from build123d import *

# Parameters (mm, degrees)
SKETCH7_R           = 50
BOSS_EXTRUDE3_DEPTH = 124.4
SKETCH8_R           = 37.5
CUT_EXTRUDE3_DEPTH  = 56
SKETCH9_R           = 32.5
CUT_EXTRUDE4_DEPTH  = 69.4
SKETCH10_W          = 250
SKETCH10_H          = 100
BOSS_EXTRUDE4_DEPTH = 15
SKETCH11_R          = 37.5
CUT_EXTRUDE5_DEPTH  = 15
SKETCH12_R          = 15
BOSS_EXTRUDE5_DEPTH = 328
LPATTERN1_COUNT     = 2
LPATTERN1_PITCH     = 180
SKETCH13_W          = 250
SKETCH13_H          = 100
BOSS_EXTRUDE6_DEPTH = 15
SKETCH15_R          = 20
CUT_EXTRUDE6_DEPTH  = 15


with BuildPart() as part:
    # Sketch7 → Boss-Extrude3 (new body)
    with BuildSketch(Plane.XY):
        with Locations((15.572802758, -20.527785454)):
            Circle(SKETCH7_R)
    extrude(amount=BOSS_EXTRUDE3_DEPTH)

    # Sketch8 → Cut-Extrude3 (cut)
    with BuildSketch(Plane.XY.offset(124.4)):
        with Locations((15.572802758, -20.527785454)):
            Circle(SKETCH8_R)
    extrude(amount=-CUT_EXTRUDE3_DEPTH, mode=Mode.SUBTRACT)

    # Sketch9 → Cut-Extrude4 (cut)
    with BuildSketch(Plane(origin=(0, 0, 0), x_dir=(-1, 0, 0), z_dir=(0, 0, -1))):
        with Locations((-15.572802758, -20.527785454)):
            Circle(SKETCH9_R)
    extrude(amount=-CUT_EXTRUDE4_DEPTH, mode=Mode.SUBTRACT)

    # Sketch10 → Boss-Extrude4 (add)
    with BuildSketch(Plane.XY.offset(124.4)):
        with Locations((15.572802758, -20.527785454)):
            Rectangle(SKETCH10_W, SKETCH10_H)
    extrude(amount=BOSS_EXTRUDE4_DEPTH)

    # Sketch11 → Cut-Extrude5 (cut)
    with BuildSketch(Plane.XY.offset(139.4)):
        with Locations((15.572802758, -20.527785454)):
            Circle(SKETCH11_R)
    extrude(amount=-CUT_EXTRUDE5_DEPTH, mode=Mode.SUBTRACT)

    # Sketch12 → Boss-Extrude5 (add)
    with BuildSketch(Plane.XY.offset(139.4)):
        with Locations((105.572802758, -20.527785454)):
            Circle(SKETCH12_R)
    boss_extrude5 = extrude(amount=BOSS_EXTRUDE5_DEPTH)

    # LPattern1: Boss-Extrude5 ×2
    with Locations(*[(-i * LPATTERN1_PITCH, 0, 0) for i in range(1, LPATTERN1_COUNT)]):
        add(boss_extrude5)

    # Sketch13 → Boss-Extrude6 (add)
    with BuildSketch(Plane.XY.offset(467.4)):
        with Locations((15.572802758, -20.527785454)):
            Rectangle(SKETCH13_W, SKETCH13_H)
    extrude(amount=BOSS_EXTRUDE6_DEPTH)

    # Sketch15 → Cut-Extrude6 (cut)
    with BuildSketch(Plane.XY.offset(482.4)):
        with Locations((15.572802758, -20.527785454)):
            Circle(SKETCH15_R)
    extrude(amount=-CUT_EXTRUDE6_DEPTH, mode=Mode.SUBTRACT)


solid = part.part
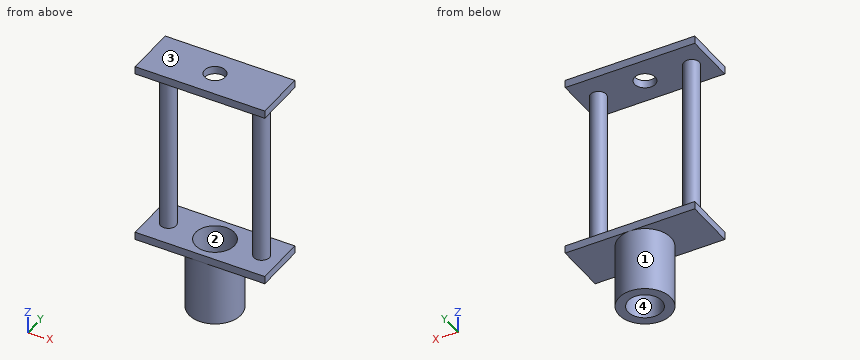
Work out the finished part from the listing and answer in its coordinate system (mm). Face numbers are marked on the shaded views. Coordinates: 2 decimals unless noted, no trailing zeros. Loops run counter-clockwise (first coordinate to the right, second up) from the corner with the lowest first, then second, coordinate; pieces in that order, holes last. Notation, with made-up numbers: (43, 34) -> (101, 34) arc R21 ccw to (101, 57) -> close; hole circle Ø2 at (40, 9.25). An arc over 180 degrees is marked (long way). Write each question's results on one line, items separated by ' | '. Start each with the question number.
1) Consider line 1 along Z through (x, y) = (-92, -19); line 2 along Z through (x, y) = (42.5, 6.5); line 3 along X through (y, z) = (-18.5, 40.5). Determine where each line is inside the solid, lowest interval first.
2) Flat-ended cylindrical pins translate along their axes: P1, Ø4, axis at x = 21, y = -49.5, coming from the -Z side; P2, Ø1.5, axis at x = -82.5, z = 424.5, coming from the +Y side; P3, Ø8, axis at y = -44.5, z = 73, coming from the +X side. Find the tip coordinate at first contact, or state that the pin passes through.
3) Find section D-D on y = 21.5. Determine the outline of the cut face in (x, z), then the cut area to 3 significant figures.
4) Find section B-B on y = -63. Determine the outline of the cut face in (x, z), then the cut area to 3 significant figures.
5) Find section C-C on z = 290. Determine the outline of the cut face in (x, y).
6) Find section A-A on x = -50.5. Determine the outline of the cut face in (y, z).
7) The mould has two halves that part along X. Classify the marked faces 1, 2, 3 and 4: pulls with the +X half, pulls with the -X half, needs draft (parallel to the pull), parting line crosses it, or undercut.
Response values:
1) line 1: z = 124.4 to 139.4, 467.4 to 482.4 | line 2: z = 0 to 139.4, 467.4 to 482.4 | line 3: x = -34.39 to -16.86, 48.01 to 65.53
2) P1: stops at z = 467.4 | P2: stops at y = -7.44 | P3: stops at x = 61.41
3) outline: (-109.43, 124.4) -> (-11.51, 124.4) -> (-11.51, 0) -> (42.66, 0) -> (42.66, 124.4) -> (140.57, 124.4) -> (140.57, 139.4) -> (-109.43, 139.4) -> close; (-109.43, 467.4) -> (140.57, 467.4) -> (140.57, 482.4) -> (-109.43, 482.4) -> close | area: 14,200 mm^2
4) outline: (-109.43, 124.4) -> (-10.81, 124.4) -> (-10.81, 0) -> (41.96, 0) -> (41.96, 124.4) -> (140.57, 124.4) -> (140.57, 139.4) -> (-109.43, 139.4) -> close; (-109.43, 467.4) -> (140.57, 467.4) -> (140.57, 482.4) -> (-109.43, 482.4) -> close | area: 14,100 mm^2
5) outline: circle Ø30 at (-74.43, -20.53); circle Ø30 at (105.57, -20.53)
6) outline: (-70.53, 124.4) -> (29.47, 124.4) -> (29.47, 139.4) -> (-70.53, 139.4) -> close; (-70.53, 467.4) -> (29.47, 467.4) -> (29.47, 482.4) -> (-70.53, 482.4) -> close
7) face 1: parting line crosses it | face 2: undercut | face 3: needs draft | face 4: undercut
